Input: part model. Units: mm. Frame: model coordinates. A direction names the side the tool comes from. Give positions to 0.01 mm unless a question says otherwise; leave off trailing zeros. Write each loop counter-clockwise with the first axis right and the second up, starting at its lowest first coordinate (ties: lowest second). Pieces come first, ordered by that corner, then holes. Notation, with made-up numbers: (-35, 3.25) -> (15, 3.25) arc R14 ccw to (15, 13.25) -> close; hole circle Ø5 at (-0.75, -6). An arc over 180 degrees is marked (long way). Return JSON: item names as keys, results as strings. Group by question number.
Item 1: Section C-C, the plane x = -1.5. Return loops of the section in (y, z), then the cut area to 3 significant figures.
Item 2: Pin query (flat end, axial travel): P1, Ø11, axis at x = 2, y = -28.5, coming from the +Z side; P2, Ø5, axis at x = 0, y = 25.4, coming from the +Z side; P3, Ø10, axis at x = 0, y = -25.4, coming from the +Z side. Return the tip coordinate at first contact, or that it passes through.
Item 3: Section A-A, the plane y = 25.4. Return loops of the section in (x, z).
Item 4: Set-up query: faces 5 (the face through (-0.878, -18.714, 8.793)), 6 (the face through (0, -1, -12.7)). Return all of +Z, -Z, +X, -X, +Y, -Y with unobstructed straight access to the full face (end or side cutting, diameter ignored); none if empty.
Item 5: Line query: line 1 (Y direction, x = 0, z = -3.25); line 2 (Y direction, x = 0, z = 10); line 3 (Z direction, x = 0.5, y = 31.5). Output: solid intervals per line, ascending. Write a range as [from, to].
Item 6: Section D-D, the plane y = -20. Return loops of the section in (x, z).
Item 7: Mould query, pull axis Y, two halves, no side actions, for faces 1 (the face through (0, -38.1, 0)), 2 (the face through (-1.462, 18.817, 8.793)), 3 (the face through (0, -30, 4.775)), 4 (the face through (0, -1, 12.7)). Classes: released by +Y, released by -Y, zero draft, split by the parting line, or undercut.
Item 8: Section B-B, the plane z = -0.5. Return loops of the section in (x, y).
from build123d import *

# Parameters (mm, degrees)
SKETCH1_W                                         = 76.2
SKETCH1_H                                         = 25.4
BOSS_EXTRUDE1_DEPTH                               = 12.7
CBORE_FOR_5_16_SOCKET_HEAD_CAP_SCREW1_D           = 8.7376
CBORE_FOR_5_16_SOCKET_HEAD_CAP_SCREW1_DEPTH       = 25.4
CBORE_FOR_5_16_SOCKET_HEAD_CAP_SCREW1_CBORE_D     = 13.4874
CBORE_FOR_5_16_SOCKET_HEAD_CAP_SCREW1_CBORE_DEPTH = 7.9248
CBORE_FOR_5_16_SOCKET_HEAD_CAP_SCREW1_TIP         = 2.625039872


with BuildPart() as part:
    # Sketch1 → Boss-Extrude1 (new, symmetric)
    with BuildSketch(Plane(origin=(0, 0, 0), x_dir=(0, 1, 0), z_dir=(0, 0, 1))):
        Rectangle(SKETCH1_W, SKETCH1_H)
    extrude(amount=BOSS_EXTRUDE1_DEPTH, both=True)

    # CBORE for 5/16 Socket Head Cap Screw1
    with Locations(Plane.XY.offset(12.7)):
        with Locations((0, -25.4), (0, 25.4)):
            CounterBoreHole(CBORE_FOR_5_16_SOCKET_HEAD_CAP_SCREW1_D / 2, CBORE_FOR_5_16_SOCKET_HEAD_CAP_SCREW1_CBORE_D / 2, CBORE_FOR_5_16_SOCKET_HEAD_CAP_SCREW1_CBORE_DEPTH, depth=CBORE_FOR_5_16_SOCKET_HEAD_CAP_SCREW1_DEPTH)
            with Locations((0, 0, -(CBORE_FOR_5_16_SOCKET_HEAD_CAP_SCREW1_DEPTH + CBORE_FOR_5_16_SOCKET_HEAD_CAP_SCREW1_TIP / 2))):  # 118° drill point
                Cone(0, CBORE_FOR_5_16_SOCKET_HEAD_CAP_SCREW1_D / 2, CBORE_FOR_5_16_SOCKET_HEAD_CAP_SCREW1_TIP, mode=Mode.SUBTRACT)


solid = part.part
Answer below:
{
 "1": {"outline": "(-38.1, -12.7) -> (-29.5, -12.7) -> (-29.5, 4.78) -> (-31.97, 4.78) -> (-31.97, 12.7) -> (-38.1, 12.7) -> close; (-21.3, -12.7) -> (21.3, -12.7) -> (21.3, 4.78) -> (18.83, 4.78) -> (18.83, 12.7) -> (-18.83, 12.7) -> (-18.83, 4.78) -> (-21.3, 4.78) -> close; (29.5, -12.7) -> (38.1, -12.7) -> (38.1, 12.7) -> (31.97, 12.7) -> (31.97, 4.78) -> (29.5, 4.78) -> close", "area": "1,440 mm2"},
 "2": {"P1": "stops at z = 12.7", "P2": "passes through", "P3": "stops at z = 4.78"},
 "3": {"outline": "(-12.7, -12.7) -> (-4.37, -12.7) -> (-4.37, 4.78) -> (-6.74, 4.78) -> (-6.74, 12.7) -> (-12.7, 12.7) -> close; (4.37, -12.7) -> (12.7, -12.7) -> (12.7, 12.7) -> (6.74, 12.7) -> (6.74, 4.78) -> (4.37, 4.78) -> close"},
 "4": {"face 5": "+Z", "face 6": "-Z, +X, -X, +Y, -Y"},
 "5": {"line 1": "y = [-38.1, -29.77], [-21.03, 21.03], [29.77, 38.1]", "line 2": "y = [-38.1, -32.14], [-18.66, 18.66], [32.14, 38.1]", "line 3": "z = [-12.7, 4.78]"},
 "6": {"outline": "(-12.7, -12.7) -> (12.7, -12.7) -> (12.7, 12.7) -> (4.04, 12.7) -> (4.04, 4.78) -> (-4.04, 4.78) -> (-4.04, 12.7) -> (-12.7, 12.7) -> close"},
 "7": {"face 1": "released by -Y", "face 2": "undercut", "face 3": "undercut", "face 4": "zero draft"},
 "8": {"outline": "(-12.7, -38.1) -> (12.7, -38.1) -> (12.7, 38.1) -> (-12.7, 38.1) -> close; hole circle Ø8.74 at (0, -25.4); hole circle Ø8.74 at (0, 25.4)"}
}
